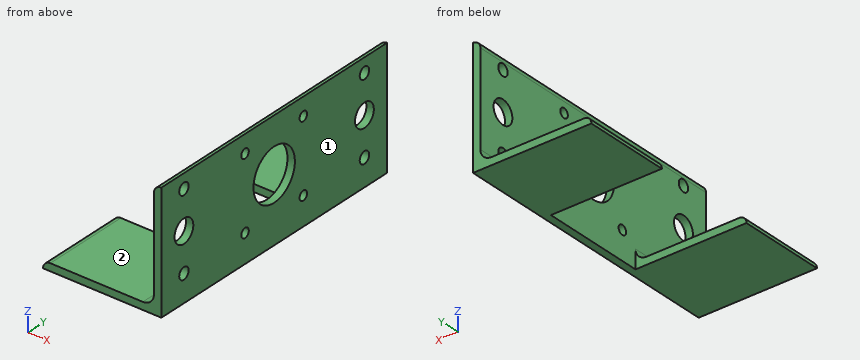
```python
from build123d import *

# Parameters (mm, degrees)
HIERRO_ANGULAR_2_X_2_X_0_125_1_DEPTH = 120
CROQUIS3_W                           = 47.625
CROQUIS3_H                           = 45
CORTAR_EXTRUIR1_DEPTH                = 10
CROQUIS4_R                           = 5
CROQUIS4_R_2                         = 2.5
CORTAR_EXTRUIR2_DEPTH                = 10
CROQUIS5_R                           = 2
CROQUIS5_R_2                         = 11
CORTAR_EXTRUIR3_DEPTH                = 3.175


with BuildPart() as part:
    # Sketch1 → Hierro angular 2 X 2 X 0.125(1) (new body)
    with BuildSketch(Plane(origin=(0, 0, 0), x_dir=(-1, 0, 0), z_dir=(0, 1, 0))):
        with BuildLine():
            Line((0, 0), (0, 50.8))
            Line((0, 50.8), (0.00508, 50.8))
            ThreePointArc((0.00508, 50.8), (2.246551928, 49.871551928), (3.175, 47.63008))
            Line((3.175, 47.63008), (3.175, 7.9375))
            ThreePointArc((3.175, 7.9375), (4.569903955, 4.569903955), (7.9375, 3.175))
            Line((7.9375, 3.175), (47.63008, 3.175))
            ThreePointArc((47.63008, 3.175), (49.871551928, 2.246551928), (50.8, 0.00508))
            Line((50.8, 0.00508), (50.8, 0))
            Line((50.8, 0), (0, 0))
        make_face()
    extrude(amount=HIERRO_ANGULAR_2_X_2_X_0_125_1_DEPTH)

    # Croquis3 → Cortar-Extruir1 (cut)
    with BuildSketch(Plane(origin=(0, 0, 0), x_dir=(-1, 0, 0), z_dir=(0, 0, -1))):
        with Locations((26.9875, 60)):
            Rectangle(CROQUIS3_W, CROQUIS3_H)
    extrude(amount=-CORTAR_EXTRUIR1_DEPTH, mode=Mode.SUBTRACT)

    # Croquis4 → Cortar-Extruir2 (cut)
    with BuildSketch(Plane.ZY.offset(3.175)):
        with Locations((28.175, 12)):
            Circle(CROQUIS4_R)
        with Locations((11.675, 12)):
            Circle(CROQUIS4_R_2)
        with Locations((44.675, 12)):
            Circle(CROQUIS4_R_2)
        with Locations((44.675, 108)):
            Circle(CROQUIS4_R_2)
        with Locations((28.175, 108)):
            Circle(CROQUIS4_R)
        with Locations((11.675, 108)):
            Circle(CROQUIS4_R_2)
    extrude(amount=-CORTAR_EXTRUIR2_DEPTH, mode=Mode.SUBTRACT)

    # Croquis5 → Cortar-Extruir3 (cut)
    with BuildSketch(Plane.ZY.offset(3.175)):
        with Locations((43.13008, 75.5)):
            Circle(CROQUIS5_R)
        with Locations((43.13008, 44.5)):
            Circle(CROQUIS5_R)
        with Locations((12.13008, 44.5)):
            Circle(CROQUIS5_R)
        with Locations((12.13008, 75.5)):
            Circle(CROQUIS5_R)
        with Locations((27.63008, 60)):
            Circle(CROQUIS5_R_2)
    extrude(amount=-CORTAR_EXTRUIR3_DEPTH, mode=Mode.SUBTRACT)


solid = part.part
```
Can you work these out from the model? Positions are in its coordinate system, mm. Face numbers are marked on the shaded views. A direction names the side the tool comes from. Give positions to 0.01 mm unless a question says otherwise; leave off trailing zeros. Loops run counter-clockwise (first coordinate to the right, second up) from the corner with the lowest first, then second, coordinate; pieces in that order, holes last. Notation, with made-up numbers: M -16,72.5 L 41,72.5 A27 cw 41,101.5 Z; hole C 54,-36 d8. An arc over 180 degrees is marked long. Use one line per item in the form item = value. Start each with the question number.
(1) On a 3-axis mill with a long thin cutter (end or side, diameter ignored), from which of +Z, -Z, +X, -X, +Y, -Y can I reach the whole of each face in a straight line? I mean the marked faces 1 and 2. Say none if no direction works.
(2) I want a section at D-D, the plane y = 108. State how many separate pieces and enclosed holes the cut face has, and give its area (3 significant figures).
(3) I want a section at B-B, the plane y = 60. Write out the boundary of the cut face in (x, z) (3 decimals).
(4) Please list where these lines run through material, in increasing order: line 1 (Z direction, x = -30.5, y = 88) (3 decimals); line 2 (X direction, y = 47, z = 19) (3 decimals); line 3 (Y direction, x = -2.5, z = 30).
(5) I'm going to push flat-ended pins straight in: P1, Ø6, axis at y = 108, z = 28.175, coming from the -X side; P2, Ø8, axis at x = -16, y = 94.5, coming from the +Z side (3 decimals); P3, Ø4, axis at y = 51.5, z = 21, coming from the -X side (3 decimals). Where does each tip first touch, or does it pass through?
(6) I want a section at C-C, the plane x = -10.5. Write out the boundary of the cut face in (y, z) (3 decimals), and give its area (3 significant figures).
(7) I want a section at A-A, the plane y = 75.5. Write out the boundary of the cut face in (x, z) (3 decimals).
Worked out:
q1.face_1 = +Z, -Z, +X, +Y, -Y
q1.face_2 = +Z, -X, +Y, -Y
q2.separate_pieces = 4
q2.enclosed_holes = 0
q2.area = 250 mm²
q3.outline = M -3.175,0 L 0,0 L 0,16.63 L -3.175,16.63 Z; M -3.175,38.63 L 0,38.63 L 0,50.8 L -0.005,50.8 A3.17 ccw -3.175,47.63 Z
q4.line_1 = 0 to 3.175
q4.line_2 = -3.175 to 0
q4.line_3 = 0 to 7.34, 16.66 to 49.26, 70.74 to 103.34, 112.66 to 120
q5.P1 = through
q5.P2 = 3.175
q5.P3 = -3.175
q6.outline = M 0,0 L 37.5,0 L 37.5,3.175 L 0,3.175 Z; M 82.5,0 L 120,0 L 120,3.175 L 82.5,3.175 Z
q6.area = 238 mm²
q7.outline = M -3.175,0 L 0,0 L 0,10.13 L -3.175,10.13 Z; M -3.175,14.13 L 0,14.13 L 0,41.13 L -3.175,41.13 Z; M -3.175,45.13 L 0,45.13 L 0,50.8 L -0.005,50.8 A3.17 ccw -3.175,47.63 Z
